Source: CAD feature listing. Evaluate the final solid. Frame: model axes, mm. A direction names the side the tool comes from. Give positions to 0.01 mm unless a question says otherwise; leave off trailing zeros. Loops run counter-clockwise (first coordinate to the right, second up) from the corner with the lowest first, then second, coordinate; pieces in that order, holes last. Notation, with made-up numbers: M 84,33 L 98,33 A28 cw 98,57 Z; hole C 20,31 d3. An arc over 180 degrees is marked long. Answer in a Markdown table with one row per item.
```python
from build123d import *

# Parameters (mm, degrees)
ESQUISSE1_R             = 7.5
ESQUISSE1_R_2           = 2.5
BOSS_EXTRU_1_DEPTH      = 12
ESQUISSE1_3_R           = 30
ESQUISSE1_3_R_2         = 6
ESQUISSE1_3_R_3         = 7.5
BOSS_EXTRU_2_DEPTH      = 3
ESQUISSE1_4_R           = 36
ESQUISSE1_4_R_2         = 30
BOSS_EXTRU_3_DEPTH      = 8.5
BOSS_EXTRU_3_DEPTH_BACK = 2


with BuildPart() as part:
    # Esquisse1 → Boss.-Extru.1 (new body)
    with BuildSketch(Plane.XY):
        Circle(ESQUISSE1_R)
        Circle(ESQUISSE1_R_2, mode=Mode.SUBTRACT)
    extrude(amount=BOSS_EXTRU_1_DEPTH)

    # Esquisse1_3 → Boss.-Extru.2 (add)
    with BuildSketch(Plane.XY):
        Circle(ESQUISSE1_3_R)
        with Locations((-16.887495374, -9.75)):
            Circle(ESQUISSE1_3_R_2, mode=Mode.SUBTRACT)
        with Locations((0, -19.5)):
            Circle(ESQUISSE1_3_R_2, mode=Mode.SUBTRACT)
        with Locations((16.887495374, -9.75)):
            Circle(ESQUISSE1_3_R_2, mode=Mode.SUBTRACT)
        with Locations((-16.887495374, 9.75)):
            Circle(ESQUISSE1_3_R_2, mode=Mode.SUBTRACT)
        Circle(ESQUISSE1_3_R_3, mode=Mode.SUBTRACT)
        with Locations((16.887495374, 9.75)):
            Circle(ESQUISSE1_3_R_2, mode=Mode.SUBTRACT)
        with Locations((0, 19.5)):
            Circle(ESQUISSE1_3_R_2, mode=Mode.SUBTRACT)
    extrude(amount=BOSS_EXTRU_2_DEPTH)

    # Esquisse1_4 → Boss.-Extru.3 (add, two sides)
    with BuildSketch(Plane.XY) as boss_extru_3_sk:
        Circle(ESQUISSE1_4_R)
        Circle(ESQUISSE1_4_R_2, mode=Mode.SUBTRACT)
    extrude(amount=BOSS_EXTRU_3_DEPTH)
    extrude(boss_extru_3_sk.sketch, amount=-BOSS_EXTRU_3_DEPTH_BACK)


solid = part.part
```
1) Material intervals for L1, parallel to Y at x = 0, z = 4.5; L2, parallel to Y at x = 0, z = 1.05; L3, parallel to Y at x = -20, z = 1.5, sorted ascending.
Reply:
| item | result |
|---|---|
| L1 | y = -36 to -30, -7.5 to -2.5, 2.5 to 7.5, 30 to 36 |
| L2 | y = -36 to -25.5, -13.5 to -2.5, 2.5 to 13.5, 25.5 to 36 |
| L3 | y = -29.93 to -14.88, -4.62 to 4.62, 14.88 to 29.93 |
2) Pin query (flat end, axial travel): pin 1 Ø12 at (x, y) = (13, -16.5) entering from -Z; pin 2 Ø19 at (x, y) = (16.89, -9.75) entering from +Z; pin 3 Ø2 at (y, z) = (13, 5.5) entering from +X; pin 4 Ø6 at (y, z) = (3, 6) entering from +X. Return the tip coordinate at first contact, or that it passes through.
Reply:
| item | result |
|---|---|
| pin 1 | stops at z = 0 |
| pin 2 | stops at z = 3 |
| pin 3 | stops at x = 33.94 |
| pin 4 | stops at x = 36 |
3) Section D-D, the plane z = 1.25. Return loops of the section in (x, y), then the cut area to 3 significant figures.
Reply:
| item | result |
|---|---|
| outline | C 0,0 d72; hole C -16.89,-9.75 d12; hole C -16.89,9.75 d12; hole C 0,-19.5 d12; hole C 0,19.5 d12; hole C 0,0 d5; hole C 16.89,-9.75 d12; hole C 16.89,9.75 d12 |
| area | 3,370 mm² |
4) Pull-direction query (X, two-part tool) for faces 4 (the flat face through (-14, 27, -2)), 5 (the cylindrical face through (-11.345, 7.452, 1.479)), 6 (the cylindrical face through (-4.686, 35.694, 3.324)); classes: released by +X, released by -X, zero draft, split by the parting line, or undercut.
Reply:
| item | result |
|---|---|
| face 4 | zero draft |
| face 5 | undercut |
| face 6 | split by the parting line |
5) Set-up query: faces 1 (the flat face through (0, -6, 0)), 2 (the flat face through (-2, 2, 12)), 3 (the cylindrical face through (-7.493, 0.33, 7.437)). Return all of +Z, -Z, +X, -X, +Y, -Y with unobstructed straight access to the full face (end or side cutting, diameter ignored); none if empty.
Reply:
| item | result |
|---|---|
| face 1 | -Z |
| face 2 | +Z, +X, -X, +Y, -Y |
| face 3 | +Z |
6) Section B-B, the plane z = 7.5. Return loops of the section in (x, y), then the cut area to 3 significant figures.
Reply:
| item | result |
|---|---|
| outline | C 0,0 d72; C 0,0 d15; hole C 0,0 d60; hole C 0,0 d5 |
| area | 1,400 mm² |
7) Section C-C, the plane x = -3.5. Return loops of the section in (y, z).
Reply:
| item | result |
|---|---|
| outline | M -35.83,-2 L -29.8,-2 L -29.8,0 L -24.37,0 L -24.37,3 L -29.8,3 L -29.8,8.5 L -35.83,8.5 Z; M -14.63,0 L 14.63,0 L 14.63,3 L 6.63,3 L 6.63,12 L -6.63,12 L -6.63,3 L -14.63,3 Z; M 24.37,0 L 29.8,0 L 29.8,-2 L 35.83,-2 L 35.83,8.5 L 29.8,8.5 L 29.8,3 L 24.37,3 Z |
8) Section A-A, the plane y = 0. Return loops of the section in (x, z).
Reply:
| item | result |
|---|---|
| outline | M -36,-2 L -30,-2 L -30,0 L -2.5,0 L -2.5,12 L -7.5,12 L -7.5,3 L -30,3 L -30,8.5 L -36,8.5 Z; M 2.5,0 L 30,0 L 30,-2 L 36,-2 L 36,8.5 L 30,8.5 L 30,3 L 7.5,3 L 7.5,12 L 2.5,12 Z |
